from build123d import *

# Parameters (mm, degrees)
SKETCH_1_W          = 47
SKETCH_1_H          = 41
EXTRUDE_1_DEPTH     = 29
SKETCH_2_W          = 7.275664065
SKETCH_2_H          = 41
CUT_EXTRUDE_1_DEPTH = 8
SKETCH_3_W          = 32.44867187
SKETCH_3_H          = 32.44867187
EXTRUDE_2_DEPTH     = 10
SKETCH_4_W          = 2.477658442
SKETCH_4_H          = 41
EXTRUDE_3_DEPTH     = 10
SKETCH_5_R          = 2.381517546
EXTRUDE_4_DEPTH     = 50
SKETCH_6_R          = 2.5
EXTRUDE_5_DEPTH     = 20
SKETCH_7_R          = 2.218731485
SKETCH_7_R_2        = 2.107008454
EXTRUDE_6_DEPTH     = 30
EXTRUDE_7_DEPTH     = 30


with BuildPart() as part:
    # Эскиз1 → Бобышка-Вытянуть1 (new body)
    with BuildSketch(Plane.XY):
        Rectangle(SKETCH_1_W, SKETCH_1_H)
    extrude(amount=EXTRUDE_1_DEPTH)

    # Эскиз2 → Вырез-Вытянуть1 (cut)
    with BuildSketch(Plane.XY.offset(29)):
        with Locations((-19.862167967, 0)):
            Rectangle(SKETCH_2_W, SKETCH_2_H)
        with Locations((19.862167967, 0)):
            Rectangle(SKETCH_2_W, SKETCH_2_H)
    extrude(amount=-CUT_EXTRUDE_1_DEPTH, mode=Mode.SUBTRACT)

    # Эскиз3 → Бобышка-Вытянуть2 (add)
    with BuildSketch(Plane.XY.offset(29)):
        Rectangle(SKETCH_3_W, SKETCH_3_H)
    extrude(amount=EXTRUDE_2_DEPTH)

    # Эскиз4 → Бобышка-Вытянуть3 (add)
    with BuildSketch(Plane.ZY.offset(23.5)):
        with Locations((11.738829221, 0)):
            Rectangle(SKETCH_4_W, SKETCH_4_H)
    extrude(amount=EXTRUDE_3_DEPTH)

    # Эскиз5 → Бобышка-Вытянуть4 (add)
    with BuildSketch(Plane.XY.offset(12.977658442)):
        with Locations(Location((-28.5, 16.509831399, 0), (0, 0, 180))):
            Circle(SKETCH_5_R)
        with Locations(Location((-28.5, -16.509831399, 0), (0, 0, 180))):
            Circle(SKETCH_5_R)
    extrude(amount=EXTRUDE_4_DEPTH)

    # Эскиз6 → Бобышка-Вытянуть5 (add)
    with BuildSketch(Plane.XY.offset(12.977658442)):
        with Locations(Location((-28.5, 5.969771762, 0), (0, 0, 180))):
            Circle(SKETCH_6_R)
        with Locations(Location((-28.5, 0, 0), (0, 0, 180))):
            Circle(SKETCH_6_R)
        with Locations(Location((-28.5, -5.977057546, 0), (0, 0, 180))):
            Circle(SKETCH_6_R)
    extrude(amount=EXTRUDE_5_DEPTH)

    # Эскиз7 → Бобышка-Вытянуть6 (add)
    with BuildSketch(Plane.XY.offset(12.977658442)):
        with Locations(Location((-28.5, 11.429883276, 0), (0, 0, 180))):
            Circle(SKETCH_7_R)
        with Locations(Location((-28.5, -11.605053901, 0), (0, 0, 180))):
            Circle(SKETCH_7_R_2)
    extrude(amount=EXTRUDE_6_DEPTH)

    # Эскиз8 → Бобышка-Вытянуть7 (add)
    with BuildSketch(Plane.XY.offset(42.977658442)):
        with BuildLine():
            Line((-23.480513429, 11.429883276), (-23.480513429, -11.605053901))
            ThreePointArc((-23.480513429, -11.605053901), (-28.5, -16.624540472), (-33.519486571, -11.605053901))
            Line((-33.519486571, -11.605053901), (-33.519486571, 11.429883276))
            ThreePointArc((-33.519486571, 11.429883276), (-28.5, 16.449369847), (-23.480513429, 11.429883276))
        make_face()
    extrude(amount=EXTRUDE_7_DEPTH)


solid = part.part
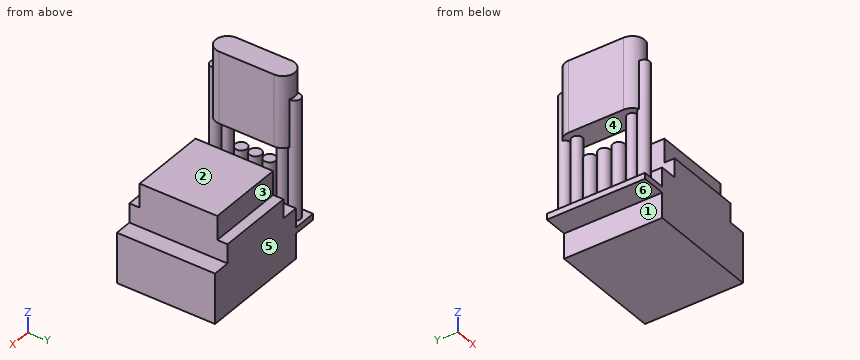
Could you check a few things on this model? Use its own coordinates, in mm. Face numbers are marked on the shaded views. A direction names the side the tool comes from. Give positions to 0.01 mm unless a question says otherwise; leave off trailing zeros. Write each loop counter-clockwise with the first axis right and the second up, starting at its lowest first coordinate (ties: lowest second). Pieces come first, ordered by that corner, then holes. Notation, with made-up numbers: (52, -7) -> (110, -7) arc R32 cw to (110, 21) -> close; hole circle Ø8 at (46, -21). An arc over 180 degrees is marked (long way). Write each question's results on one line, items separated by ' | '. Start each with the question number.
Q1. I'm going to push flat-ended pins straight in: pin 1 Ø10 at (y, z) = (-10.5, 28) entering from -X; pin 2 Ø18.5 at (y, z) = (1.5, 51) entering from +X; pin 3 Ø8 at (x, z) = (-5, 35) entering from +Y; pin 4 Ø3 at (x, y) = (-11, 14) entering from -Z. Where does each tip first touch, or does it pass through?
Q2. Suppose I cut it at D-D, the plane z = 58.5. List the corners of the cut face in (x, y) for me.
Q3. Suppose I cut it at B-B, the plane y = -7. List the corners of the cut face in (x, z) for me, and give its area (3 significant figures).
Q4. Suppose I cut it at A-A, the plane x = -1.5. List the corners of the cut face in (y, z) for me.
Q5. Which directions (+Z, -Z, +X, -X, +Y, -Y) give clear straight access to the entire face, cutting with the end or side of a thin tool? Please do the marked faces 1, 2 and 3.
Q6. I need wall thicknesses on probe 1 along Z at (x, y) = (-27, 6.5); probe 2 along X at (y, z) = (5.5, 51.5); probe 3 along X at (y, z) = (13, 16.5). Which ranges of each line are inside material? Lowest first, please.
Q7. Suppose I cut it at C-C, the plane z = 18. List the corners of the cut face in (x, y) for me, and give its area (3 significant figures).
Q8. We'd pull the mould along Z, two halves only. Please class the marked faces 4, 5 and 6: +Z half, -Z half, draft (parallel to the pull), parting line (faces both ways), or undercut.
Outcome:
1) pin 1: x = -31 | pin 2: x = -23.48 | pin 3: y = 16.22 | pin 4: z = 0
2) outline: (-33.52, -11.61) arc R5.02 ccw to (-30.84, -16.05) arc R2.38 ccw (long way) to (-26.16, -16.05) arc R5.02 ccw to (-23.48, -11.61) -> (-23.48, 11.43) arc R5.02 ccw to (-26.2, 15.89) arc R2.38 ccw (long way) to (-30.8, 15.89) arc R5.02 ccw to (-33.52, 11.43) -> close
3) outline: (-33.52, 42.98) -> (-23.48, 42.98) -> (-23.48, 72.98) -> (-33.52, 72.98) -> close; (-33.5, 10.5) -> (-23.5, 10.5) -> (-23.5, 0) -> (23.5, 0) -> (23.5, 21) -> (16.22, 21) -> (16.22, 39) -> (-16.22, 39) -> (-16.22, 21) -> (-23.5, 21) -> (-23.5, 12.98) -> (-26.22, 12.98) -> (-26.22, 32.98) -> (-30.78, 32.98) -> (-30.78, 12.98) -> (-33.5, 12.98) -> close | area: 1,990 mm2
4) outline: (-20.5, 0) -> (20.5, 0) -> (20.5, 29) -> (16.22, 29) -> (16.22, 39) -> (-16.22, 39) -> (-16.22, 29) -> (-20.5, 29) -> close
5) face 1: -Z, -X, +Y, -Y | face 2: +Z, +X, +Y, -Y | face 3: +Z, +X, +Y
6) probe 1: 10.5 to 32.98, 42.98 to 72.98 | probe 2: -33.52 to -23.48 | probe 3: -30.07 to -26.93, -23.5 to 23.5
7) outline: circle Ø5 at (-28.5, -5.98); circle Ø5 at (-28.5, 0); circle Ø5 at (-28.5, 5.97); circle Ø4.76 at (-28.5, -16.51); circle Ø4.76 at (-28.5, 16.51); circle Ø4.44 at (-28.5, 11.43); circle Ø4.21 at (-28.5, -11.61); (-23.5, -20.5) -> (23.5, -20.5) -> (23.5, 20.5) -> (-23.5, 20.5) -> close | area: 2,050 mm2
8) face 4: undercut | face 5: draft | face 6: -Z half
